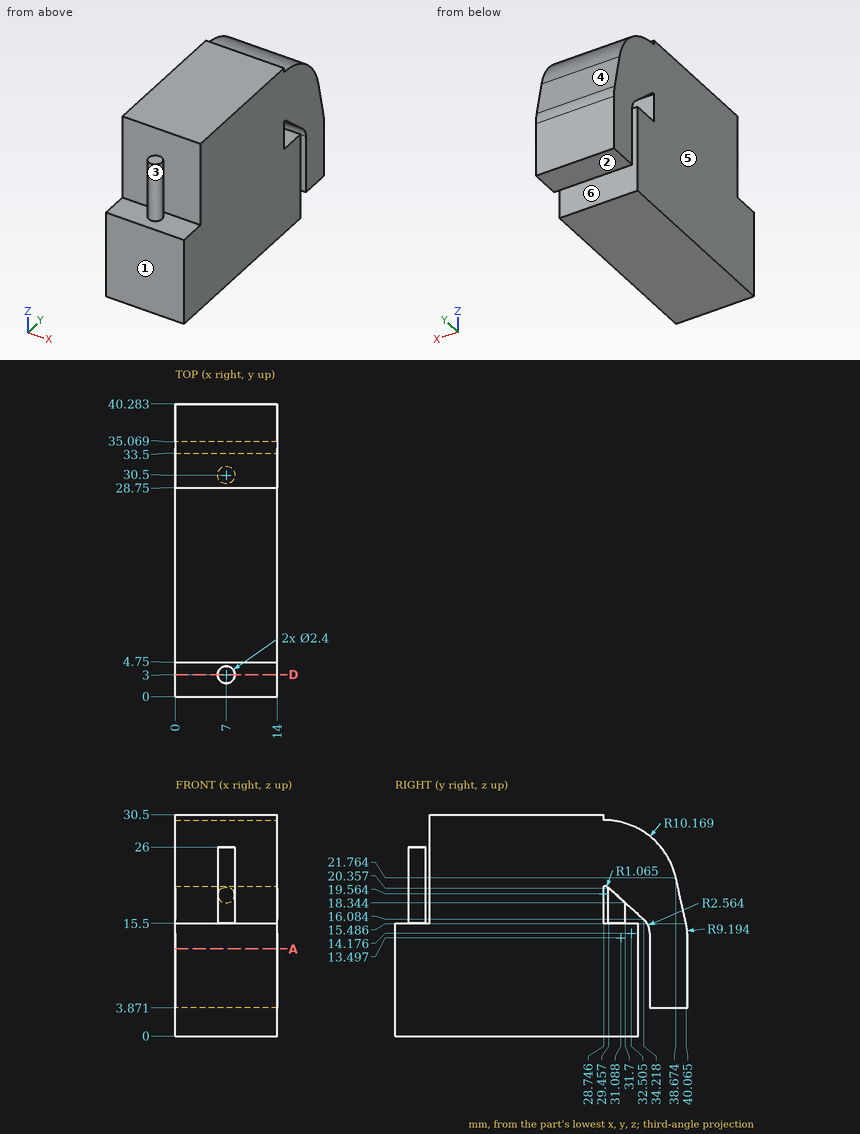
Check sheet for the drawn part. Datum: minimum x, y, z corner. Units: mm. A direction names the side the tool comes from. Round coordinates to 2 decimals unless told otherwise and drop trailing zeros. Order: outer loops, then holes, each group sorted by start corner. A loop starts at its lowest first (then second) coordinate and runs counter-clockwise, first axis right, second up. Notation, with made-up numbers: (-1, 18) -> (34, 18) arc R15 ccw to (34, 45) -> close; hole circle Ø1 at (-22.75, 84.25). An arc over 180 degrees is marked (long way). Put each result on its own line as item: value.
1) Material ranges on line 1 (Y direction, x = 11.5, z = 8); line 2 (X direction, y = 3, z = 24.5); line 3 (Y direction, x = 3, z = 14.5), recorded low to high.
Final values:
line 1: y = 0 to 33.5, 35.07 to 40.28
line 2: x = 5.8 to 8.2
line 3: y = 0 to 33.5, 35.05 to 40.23
2) Depth check by flat-ended pin: pin 1 (7 mm diameter, centred on x = 8, z = 26, fed in from -Y); pin 2 (5 mm diameter, centred on x = 9.5, y = 34, fed in from +Z); pin 3 (1.5 mm diameter, centred on x = 9, y = 10.5, fed in from -Z); pin 4 (1.6 mm diameter, centred on x = 9, y = 36.5, fed in from -Z). Enter the tip coordinate at first touch or a pass-through.
Final values:
pin 1: stops at y = 1.8
pin 2: stops at z = 29.35
pin 3: stops at z = 0
pin 4: stops at z = 3.87
3) Section check A-A (z = 12). Record the cut outline in (x, y), then the cut area to 3 significant figures.
Final values:
outline: (0, 0) -> (14, 0) -> (14, 33.5) -> (0, 33.5) -> close; (0, 35.07) -> (14, 35.07) -> (14, 40.28) -> (0, 40.28) -> close
area: 542 mm^2
4) Mould release check, pull along Y, two halves, no side actions. Record for the marked faces 4, 5 and 6: +Y half, -Y half, draft (parallel to the pull), parting line (faces both ways), or undercut.
Final values:
face 4: +Y half
face 5: draft
face 6: undercut
5) Section check D-D (y = 3). Record the cut outline in (x, z).
Final values:
outline: (0, 0) -> (14, 0) -> (14, 15.5) -> (8.2, 15.5) -> (8.2, 26) -> (5.8, 26) -> (5.8, 15.5) -> (0, 15.5) -> close
6) Set-up check for the marked faces 1, 2 and 3: record each of +Z, -Z, +X, -X, +Y, -Y from which the full face is reachable in a straight line by a thin tool's end or side.
Final values:
face 1: +Z, -Z, +X, -X, -Y
face 2: -Z, +X, -X, +Y
face 3: +Z
